from build123d import *

# Parameters (mm, degrees)
SM_BASE_FLANGE_1_DEPTH      = 40
CHAMFER_1_SIZE              = 5
CUT_EXTRUDE_1_DEPTH         = 258.126428047
CUT_EXTRUDE_2_DEPTH         = 256.076459125
HOLE_START                  = -3
HOLE_WIZARD_6_2_6_2_1_DEPTH = 3


# Read off the part's stored shape, not the designer's step: Ø6.2 (6.2) 直径槽口1
# Sheet-metal steps are written as plain solids
with BuildPart() as part:
    # Sketch 2 → 基体-法兰1 (new, symmetric)
    with BuildSketch(Plane.XY):
        with BuildLine():
            Line((0, 245), (0, 4.5))
            ThreePointArc((0, 4.5), (-1.318019485, 1.318019485), (-4.5, 0))
            Line((-4.5, 0), (-70, 0))
            Line((-70, 0), (-70, 3))
            Line((-70, 3), (-4.5, 3))
            ThreePointArc((-4.5, 3), (-3.439339828, 3.439339828), (-3, 4.5))
            Line((-3, 4.5), (-3, 245))
            Line((-3, 245), (0, 245))
        make_face()
    extrude(amount=SM_BASE_FLANGE_1_DEPTH, both=True)

    # 倒角1
    chamfer_1_edges = [part.edges().sort_by_distance(p)[0] for p in [
        (-1.5, 245, 40),
        (-70, 1.5, 40),
        (-1.5, 245, -40),
        (-70, 1.5, -40),
    ]]
    chamfer(chamfer_1_edges, length=CHAMFER_1_SIZE)

    # 草图7 → 切除-拉伸1 (cut, through all)
    with BuildSketch(Plane.ZY.offset(3)):
        with BuildLine():
            Line((-28.9, 237), (-28.9, 207))
            ThreePointArc((-28.9, 207), (-32, 203.9), (-35.1, 207))
            Line((-35.1, 207), (-35.1, 237))
            ThreePointArc((-35.1, 237), (-32, 240.1), (-28.9, 237))
        make_face()
    cut_extrude_1 = extrude(amount=-CUT_EXTRUDE_1_DEPTH, mode=Mode.SUBTRACT)

    # 草图10 → 切除-拉伸2 (cut, through all)
    with BuildSketch(Plane(origin=(0, 3, 0), x_dir=(1, 0, 0), z_dir=(0, 1, 0))):
        with BuildLine():
            Line((-55, 35.1), (-30, 35.1))
            ThreePointArc((-30, 35.1), (-26.9, 32), (-30, 28.9))
            Line((-30, 28.9), (-55, 28.9))
            ThreePointArc((-55, 28.9), (-58.1, 32), (-55, 35.1))
        make_face()
    cut_extrude_2 = extrude(amount=-CUT_EXTRUDE_2_DEPTH, mode=Mode.SUBTRACT)

    # 镜向1: 切除-拉伸1, 切除-拉伸2 across plane
    add(cut_extrude_1.mirror(Plane.XY), mode=Mode.SUBTRACT)
    add(cut_extrude_2.mirror(Plane.XY), mode=Mode.SUBTRACT)

    # Ø6.2 (6.2) 直径槽口1 outline → Ø6.2 (6.2) 直径槽口1 (cut)
    with BuildSketch(Plane.YZ.offset(HOLE_START)):
        with BuildLine():
            ThreePointArc((169.9, -35.1), (173, -32), (169.9, -28.9))
            Line((169.9, -28.9), (146.1, -28.9))
            ThreePointArc((146.1, -28.9), (143, -32), (146.1, -35.1))
            Line((146.1, -35.1), (169.9, -35.1))
        make_face()
        with BuildLine():
            ThreePointArc((169.9, 28.9), (173, 32), (169.9, 35.1))
            Line((169.9, 35.1), (146.1, 35.1))
            ThreePointArc((146.1, 35.1), (143, 32), (146.1, 28.9))
            Line((146.1, 28.9), (169.9, 28.9))
        make_face()
    extrude(amount=HOLE_WIZARD_6_2_6_2_1_DEPTH, mode=Mode.SUBTRACT)


solid = part.part
The listing builds one solid part. Answer for the finished solid, in the listing's coordinates (mm). A direction names the side the tool comes from. Give positions to 0.01 mm unless a question says otherwise; leave off trailing zeros. Loops run counter-clockwise (first coordinate to the right, second up) from the corner with the lowest first, then second, coordinate; pieces in that order, holes last. Notation, with made-up numbers: (53, 61.25) - (111, 61.25) arc R34 cw to (111, 100.25) - close; hole circle Ø2 at (-39, 1.5). An arc over 180 degrees is marked (long way). Answer as a JSON object with one key per item and string values.
1. Flat-ended cylindrical pins translate along their axes: pin 1 Ø8 at (y, z) = (181.5, -18) entering from +X; pin 2 Ø3 at (x, z) = (-35.5, -25.5) entering from +Y. Find the tip coordinate at first contact, or state that the pin passes through.
Determined:
{"pin 1": "x = 0", "pin 2": "y = 3"}
2. For faces 1 (the flat face through (-2, 243, 37)), 2 (the flat face through (-3, 123, 1)), determine the directions among +Z, -Z, +X, -X, +Y, -Y from which every point of the face is accessible in a straight line to the end or side of a thin tool.
Determined:
{"face 1": "+Z, +X, -X, +Y", "face 2": "+Z, -Z, -X, +Y"}
3. A cutting plane is placed at C-C (z = 6). Write down the section's boundary in (x, y).
Determined:
{"outline": "(-70, 0) - (-4.5, 0) arc R4.5 ccw to (0, 4.5) - (0, 245) - (-3, 245) - (-3, 4.5) arc R1.5 cw to (-4.5, 3) - (-70, 3) - close"}
4. A cutting plane is placed at D-D (x = -11.5). Write down the section's boundary in (y, z).
Determined:
{"outline": "(0, -40) - (3, -40) - (3, 40) - (0, 40) - close"}
5. A cutting plane is placed at B-B (z = -32). Write down the section's boundary in (x, y), then the cut area to 3 significant figures.
Determined:
{"outline": "(-70, 0) - (-58.1, 0) - (-58.1, 3) - (-70, 3) - close; (-26.9, 0) - (-4.5, 0) arc R4.5 ccw to (0, 4.5) - (0, 143) - (-3, 143) - (-3, 4.5) arc R1.5 cw to (-4.5, 3) - (-26.9, 3) - close; (-3, 173) - (0, 173) - (0, 203.9) - (-3, 203.9) - close; (-3, 240.1) - (0, 240.1) - (0, 245) - (-3, 245) - close", "area": "640 mm²"}
6. A cutting plane is placed at A-A (x = -45.5). Write down the section's boundary in (y, z).
Determined:
{"outline": "(0, -40) - (3, -40) - (3, -35.1) - (0, -35.1) - close; (0, -28.9) - (3, -28.9) - (3, 28.9) - (0, 28.9) - close; (0, 35.1) - (3, 35.1) - (3, 40) - (0, 40) - close"}
7. Find the intervals of material crossed by L1, parallel to X at y = 89, z = 10.5; L2, parallel to Y at x = -38, z = 6, in increasing order. Write a range as [from, to].
Determined:
{"L1": "[-3, 0]", "L2": "[0, 3]"}
